The figure shows three views and two pictorial views of one solid part (mm, origin at its lowest corner). Answer the questions. Coordinates: 2 decimals unless noted, no trailing zeros. Write each loop counter-clockwise with the first axis right and the second up, starting at its lowest first coordinate (ties: lowest second). Pieces come first, ordered by that corner, then holes.
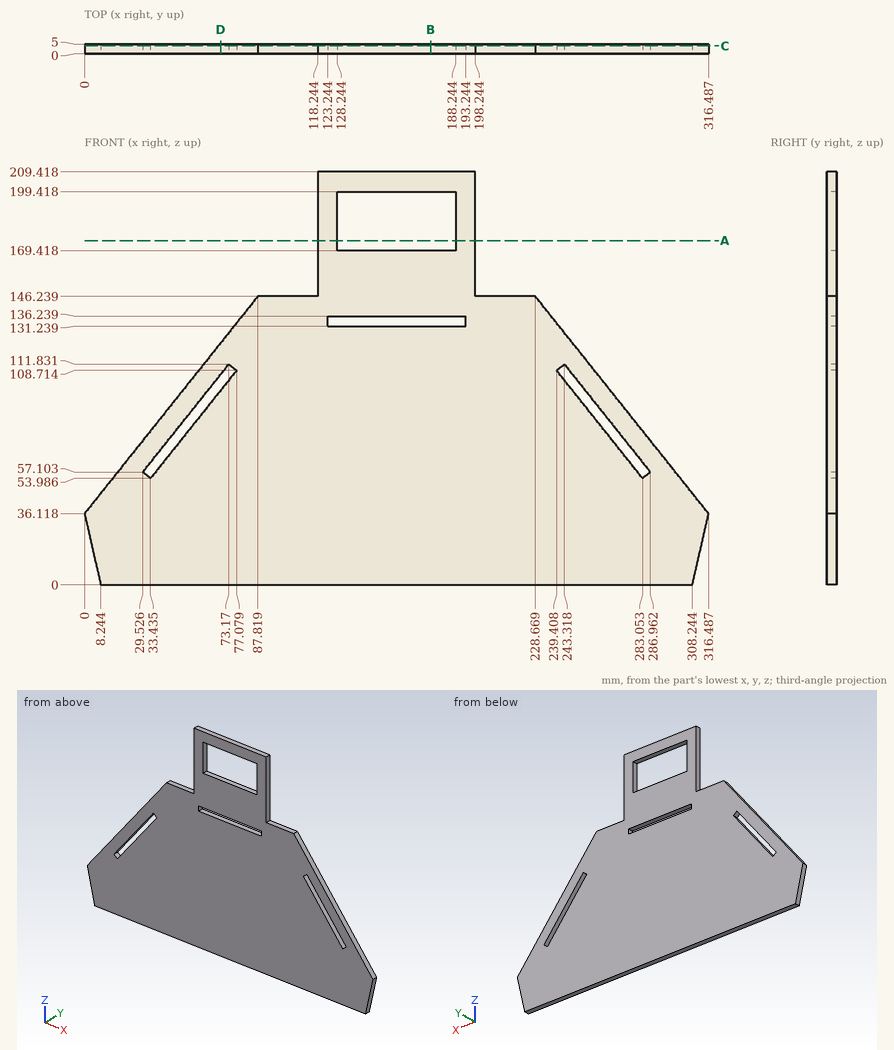
Q1. Find the intervals of material crossed by probe 1 along Z at (x, y) = (143.5, 4.4); probe 2 along X at (y, z) = (4.55, 187); probe 3 along X at (y, z) = (3.8, 108) (1 decimal), in increasing order.
Answers below:
probe 1: z = 0 to 131.24, 136.24 to 169.42, 199.42 to 209.42
probe 2: x = 118.24 to 128.24, 188.24 to 198.24
probe 3: x = 57.3 to 70.1, 76.5 to 240, 246.4 to 259.2
Q2. The part is cut by section A-A, the plane z = 174.5. Write down the section's boundary in (x, y).
Answers below:
outline: (118.24, 0) - (128.24, 0) - (128.24, 5) - (118.24, 5) - close; (188.24, 0) - (198.24, 0) - (198.24, 5) - (188.24, 5) - close
Q3. The part is cut by section D-D, the plane x = 69. Write down the section's boundary in (y, z), then the cut area to 3 significant figures.
Answers below:
outline: (0, 0) - (5, 0) - (5, 98.58) - (0, 98.58) - close; (0, 106.6) - (5, 106.6) - (5, 122.64) - (0, 122.64) - close
area: 573 mm2
Q4. Given pin 1 (2.5 mm diameter, centred on y = 3, z = 184.5, fed in from -X); pin 2 (1.5 mm diameter, centred on y = 1.5, z = 134, fed in from +X); pin 3 (1.5 mm diameter, centred on x = 114, y = 1, fed in from +Z), each flat-ended and moving along its own axis, determine where each tip first touches the part or whether it passes through.
Answers below:
pin 1: stops at x = 118.24
pin 2: stops at x = 239.03
pin 3: stops at z = 146.24
Q5. The part is cut by section C-C, the plane y = 4. Write down the section's boundary in (x, z) (1 decimal).
Answers below:
outline: (0, 36.1) - (8.2, 0) - (308.2, 0) - (316.5, 36.1) - (228.7, 146.2) - (198.2, 146.2) - (198.2, 209.4) - (118.2, 209.4) - (118.2, 146.2) - (87.8, 146.2) - close; hole (29.5, 57.1) - (33.4, 54) - (77.1, 108.7) - (73.2, 111.8) - close; hole (123.2, 131.2) - (193.2, 131.2) - (193.2, 136.2) - (123.2, 136.2) - close; hole (128.2, 169.4) - (188.2, 169.4) - (188.2, 199.4) - (128.2, 199.4) - close; hole (239.4, 108.7) - (283.1, 54) - (287, 57.1) - (243.3, 111.8) - close
Q6. The part is cut by section B-B, the plane x = 175.5. Write down the section's boundary in (y, z).
Answers below:
outline: (0, 0) - (5, 0) - (5, 131.24) - (0, 131.24) - close; (0, 136.24) - (5, 136.24) - (5, 169.42) - (0, 169.42) - close; (0, 199.42) - (5, 199.42) - (5, 209.42) - (0, 209.42) - close
